from build123d import *

# Parameters (mm, degrees)
SKETCH2_W          = 152.4
SKETCH2_H          = 28.575
BASE_FLANGE1_DEPTH = 3.175
EDGE_FLANGE1_DEPTH = 28.575
CUT_EXTRUDE1_START = -3.175
CUT_EXTRUDE1_DEPTH = 167.563083351


# Sheet-metal steps are written as plain solids
with BuildPart() as part:
    # Sketch2 → Base-Flange1 (new body)
    with BuildSketch(Plane.XY):
        Rectangle(SKETCH2_W, SKETCH2_H)
    extrude(amount=BASE_FLANGE1_DEPTH)

    # Edge-Flange1 section (across the edge) → Edge-Flange1 (add)
    with BuildSketch(Plane(origin=(77.2, -14.2875, 3.175), x_dir=(-1, 0, 0), z_dir=(0, 1, 0))):
        with BuildLine():
            Line((-3.175, 1), (-3.175, 41.275))
            Line((-3.175, 41.275), (0, 41.275))
            Line((0, 41.275), (0, 1))
            ThreePointArc((0, 1), (0.292893219, 0.292893219), (1, 0))
            Line((1, 0), (1, -3.175))
            ThreePointArc((1, -3.175), (-1.952170811, -1.952170811), (-3.175, 1))
        make_face()
    edge_flange1 = extrude(amount=EDGE_FLANGE1_DEPTH)

    # Sketch10 → Cut-Extrude1 (cut)
    with BuildSketch(Plane(origin=(80.375, 0, 0), x_dir=(0, 0, -1), z_dir=(1, 0, 0)).offset(CUT_EXTRUDE1_START)):
        Polygon((-4.175, 14.2875), (-44.45, -14.2875), (-44.45, 14.2875), align=None)
    cut_extrude1 = extrude(amount=CUT_EXTRUDE1_DEPTH, mode=Mode.SUBTRACT)

    # Mirror1: Edge-Flange1, Cut-Extrude1 across plane
    add(edge_flange1.mirror(Plane(origin=(0, 0, 0), x_dir=(0, 0, 1), z_dir=(1, 0, 0))))
    add(cut_extrude1.mirror(Plane(origin=(0, 0, 0), x_dir=(0, 0, 1), z_dir=(1, 0, 0))), mode=Mode.SUBTRACT)


solid = part.part
Source: CAD feature listing. Evaluate the final solid. Frame: model axes, mm. A direction names the side the tool comes from. Round coordinates to 2 decimals unless told otherwise and drop trailing zeros. Loops run counter-clockwise (first coordinate to the right, second up) from the corner with the lowest first, then second, coordinate; pieces in that order, holes last. Notation, with made-up numbers: M -18,58 L 1,58 A19 ccw 1,76 Z; hole C 58,38 d5. An arc over 180 degrees is marked long. Return JSON: item names as keys, results as strings. Group by question number.
1. Mould query, pull axis X, two halves, no side actions, for faces 3 (the face through (77.2, -7, 16)), 4 (the face through (1, 14.288, 2)), 5 (the face through (-77.2, -7, 16)), 6 (the face through (-80.375, -3, 20)). Classes: released by +X, released by -X, zero draft, split by the parting line, or undercut.
2. Section query D-D on z = 30. Output: boundary loops of the cut face in (x, y) (1 decimal).
3. Section query A-A on z = 38.5. Output: boundary loops of the cut face in (x, y) (1 decimal), and give its area (3 significant figures).
4. Material intervals for line 1 along X through (y, z) = (-11.75, 19.5) (3 decimals); line 2 along Z through (x, y) = (63, -6.5) (3 decimals); line 3 along X through (y, z) = (10.5, 2.5), sorted ascending. Write a range as from..to.
5. Pin query (flat end, axial travel): pin 1 (8 mm diameter, centred on x = 26.5, y = 3.5, fed in from +Z) (3 decimals). Return the tip coordinate at first contact, or that it passes through.
6. Section query B-B on y = 7.5. Output: boundary loops of the cut face in (x, z) (3 decimals), and give its area (3 significant figures).
7. Reachability of faces 1 (the face through (-1, 0, 0)), 2 (the face through (-1, 0, 3.175)) from +Z, -Z, +X, -X, +Y, -Y: full face, straight path, thin tool, end or side. Return the list, or none.
8. Section query C-C on x = 28. Output: boundary loops of the cut face in (y, z) (1 decimal).
Checks:
{
 "1": {"face 3": "undercut", "face 4": "zero draft", "face 5": "undercut", "face 6": "released by -X"},
 "2": {"outline": "M -80.4,-14.3 L -77.2,-14.3 L -77.2,-4 L -80.4,-4 Z; M 77.2,-14.3 L 80.4,-14.3 L 80.4,-4 L 77.2,-4 Z"},
 "3": {"outline": "M -80.4,-14.3 L -77.2,-14.3 L -77.2,-10.1 L -80.4,-10.1 Z; M 77.2,-14.3 L 80.4,-14.3 L 80.4,-10.1 L 77.2,-10.1 Z", "area": "26.8 mm²"},
 "4": {"line 1": "x = -80.375..-77.2, 77.2..80.375", "line 2": "z = 0..3.175", "line 3": "x = -80.02..80.02"},
 "5": {"pin 1": "stops at z = 3.175"},
 "6": {"outline": "M -80.375,4.175 A4.175 ccw -76.2,0 L 76.2,0 A4.175 ccw 80.375,4.175 L 80.375,13.742 L 77.2,13.742 L 77.2,4.175 A1 cw 76.2,3.175 L -76.2,3.175 A1 cw -77.2,4.175 L -77.2,13.742 L -80.375,13.742 Z", "area": "570 mm²"},
 "7": {"face 1": "-Z, +X, -X, +Y, -Y", "face 2": "+Z, +Y, -Y"},
 "8": {"outline": "M -14.3,0 L 14.3,0 L 14.3,3.2 L -14.3,3.2 Z"}
}
